Read the model definition and answer for the solid it produces. Units are mm, in the model's axes. A direction names the side the tool comes from. Coordinates: 2 decimals unless noted, no trailing zeros. Loops run counter-clockwise (first coordinate to the right, second up) from the corner with the lowest first, then second, coordinate; pieces in that order, holes last. Notation, with made-up numbers: M 77.25,30.5 L 86.25,30.5 A23 cw 86.25,40.5 Z; hole C -21.75,50 d6. An arc over 180 degrees is marked long. Put each result on its own line as item: value.
Autodesk Inventor part; units mm, degrees
ref_plane "YZ Plane" through (0, 0, 0) normal (1, 0, 0) x (0, 1, 0)
ref_plane "XZ Plane" through (0, 0, 0) normal (0, 1, 0) x (-1, 0, 0)
ref_plane "XY Plane" through (0, 0, 0) normal (0, 0, 1) x (1, 0, 0)
sketch "Sketch1" plane through (0, 0, 0) normal (0, 0, 1) x (1, 0, 0)
  circle A0 centre (-150, 0) radius 225 construction
  line L0 (0, 0) -> (0, 132.2876)
  line L1 (0, 132.2876) -> (17.7086, 149.9961)
  line L2 (0, 132.2876) -> (25.0437, 132.2876) construction
  arc A1 (75, 0) -> (17.7086, 149.9961) centre (-150, 0) ccw
  line L3 (75, 0) -> (25, 0)
  line L4 (25, 0) -> (17.5, 0)
  line L5 (0, 0) -> (7.5, 0)
  line L6 (7.5, 0) -> (7.5, -10)
  line L7 (7.5, -10) -> (17.5, -10)
  line L8 (17.5, -10) -> (17.5, 0)
  circle A2 centre (-150, 0) radius 200 construction
  dimension "d0" = 75
  dimension "d1" = 450
  dimension "d3" = 45
  dimension "d37" = 50
  dimension "d38" = 7.5
  dimension "d39" = 7.5
  dimension "d40" = 10
  dimension "d41" = 25
extrude "Extrusion1" add sketch "Sketch1" along normal blind 15
sketch "Sketch2" plane through (0, 0, 15) normal (0, 0, 1) x (1, 0, 0)
  circle A0 centre (58.5066, 25) radius 2.5
  circle A1 centre (56.1901, 39.8201) radius 2.5
  line L0 (0, 132.2876) -> (0, 0)
  line L1 (0, 0) -> (7.5, 0)
  line L2 (7.5, 0) -> (7.5, -10)
  line L3 (7.5, -10) -> (17.5, -10)
  line L4 (17.5, -10) -> (17.5, 0)
  line L5 (17.5, 0) -> (75, 0)
  arc A2 (75, 0) -> (17.7086, 149.9961) centre (-150, 0) ccw
  line L6 (17.7086, 149.9961) -> (0, 132.2876)
  arc A3 (59.4636, 15) -> (16.6742, 127.7486) centre (-150, 0) ccw construction
  line L7 (59.4636, 15) -> (17.5, 15) construction
  line L8 (17.5, 15) -> (15, 15) construction
  line L9 (15, 15) -> (15, 126.0744) construction
  line L10 (15, 126.0744) -> (16.6742, 127.7486) construction
  circle A4 centre (11.959, 133.676) radius 2.5
  circle A5 centre (-150, 0) radius 225 construction
  circle A6 centre (-150, 0) radius 210 construction
  dimension "d6" = 5
  dimension "d7" = 5
  dimension "d8" = 15
  dimension "d10" = 25
  dimension "d42" = 15
  dimension "d43" = 5
  dimension "d45" = 450
  dimension "d46" = 15
  dimension "d49" = 7.4745
extrude "Extrusion2" cut sketch "Sketch2" against normal through all contours A0 | A1 | A4
sketch "Sketch5" plane through (0, 0, 15) normal (0, 0, 1) x (1, 0, 0)
  line L0 (5, 137.2876) -> (12.0711, 130.2165)
  line L1 (5, 137.2876) -> (15, 137.2876) construction
  line L2 (12.0711, 130.2165) -> (15.6066, 133.752)
  line L3 (15.6066, 133.752) -> (8.5355, 140.8231)
  line L4 (8.5355, 140.8231) -> (5, 137.2876)
  line L5 (17.7086, 149.9961) -> (0, 132.2876)
  point P0 (0, 0)
  dimension "d29" = 10
  dimension "d30" = 45
  dimension "d31" = 5
  dimension "d32" = 10
  dimension "d33" = 90
  dimension "d34" = 5
extrude "Extrusion3" cut sketch "Sketch5" against normal through all
thread "Thread1"
thread "Thread2"
thread "Thread3"
sketch "Sketch6" plane through (0, 0, 15) normal (0, 0, 1) x (1, 0, 0)
  line L0 (0, 107.2876) -> (20, 107.2876) construction
  line L1 (20, 107.2876) -> (20, 57.2876) construction
  line L2 (20, 57.2876) -> (0, 57.2876) construction
  line L3 (0, 57.2876) -> (0, 107.2876) construction
  line L4 (8.5355, 140.8231) -> (15.6066, 133.752) construction
  line L5 (15.6066, 133.752) -> (12.0711, 130.2165) construction
  line L6 (9.7164, 132.5711) -> (5, 137.2876) construction
  line L7 (5, 137.2876) -> (0, 132.2876) construction
  line L8 (0, 132.2876) -> (0, 0) construction
  line L9 (0, 0) -> (7.5, 0) construction
  line L10 (7.5, 0) -> (7.5, -10) construction
  line L11 (7.5, -10) -> (17.5, -10) construction
  line L12 (17.5, -10) -> (17.5, 0) construction
  line L13 (17.5, 0) -> (75, 0) construction
  arc A0 (75, 0) -> (17.7086, 149.9961) centre (-150, 0) ccw construction
  line L14 (17.7086, 149.9961) -> (8.5355, 140.8231) construction
  arc A1 (9.7164, 132.5711) -> (10.8542, 131.4334) centre (11.959, 133.676) ccw construction
  circle A2 centre (58.5066, 25) radius 2.5 construction
  circle A3 centre (56.1901, 39.8201) radius 2.5 construction
  circle A4 centre (10, 92.2876) radius 2.5
  circle A5 centre (10, 72.2876) radius 2.5
  line L15 (0, 132.2876) -> (0, 0)
  line L16 (12.0711, 130.2165) -> (10.8542, 131.4334)
  dimension "d50" = 20
  dimension "d51" = 50
  dimension "d52" = 25
  dimension "d53" = 5
  dimension "d54" = 5
  dimension "d55" = 20
  dimension "d56" = 15
  dimension "d57" = 10
extrude "Extrusion4" cut sketch "Sketch6" against normal through all
thread "Thread4"
thread "Thread5"
sketch "Sketch8" plane through (0, 0, 0) normal (0, 0, -1) x (-1, 0, 0)
  line L0 (0, 132.2876) -> (0, 0)
  line L1 (0, 107.2876) -> (-20, 107.2876)
  line L2 (-20, 107.2876) -> (-20, 57.2876)
  line L3 (-20, 57.2876) -> (0, 57.2876)
  line L4 (0, 57.2876) -> (0, 107.2876)
  dimension "d69" = 20
  dimension "d70" = 50
  dimension "d71" = 25
extrude "Extrusion6" cut sketch "Sketch8" against normal blind 5
properties part number "CP001" material "ABS Plastic"
1) Find section D-D, the plane x = 51.5. Write down the section's boundary in (y, z).
Answer list:
outline: M 0,0 L 100.11,0 L 100.11,15 L 0,15 Z
2) Given pin 1 Ø2.5 at (x, z) = (5.5, 2.5) entering from -Y; pin 2 Ø4 at (x, y) = (10, 72.29) entering from +Z; pin 3 Ø2 at (x, z) = (55.5, 7.5) entering from +Y; pin 4 Ø2.5 at (y, z) = (81.5, 3.5) entering from -X, each flat-ended and moving along its own axis, determine where each tip first touches the part or whether it passes through.
Answer list:
pin 1: stops at y = 0
pin 2: passes through
pin 3: stops at y = 93.83
pin 4: stops at x = 20
3) Find section A-A, the plane y = 25. Write down the section's boundary in (x, z), plus the area to 3 significant figures.
Answer list:
outline: M 0,0 L 56.01,0 L 56.01,15 L 0,15 Z; M 61.01,0 L 73.61,0 L 73.61,15 L 61.01,15 Z
area: 1,030 mm^2
4) Find section B-B, the plane z = 2.25. Write down the section's boundary in (x, y).
Answer list:
outline: M 0,0 L 7.5,0 L 7.5,-10 L 17.5,-10 L 17.5,0 L 75,0 A225 ccw 17.71,150 L 8.54,140.82 L 15.61,133.75 L 12.07,130.22 L 10.85,131.43 A2.5 cw 9.72,132.57 L 5,137.29 L 0,132.29 L 0,107.29 L 20,107.29 L 20,57.29 L 0,57.29 Z; hole C 56.19,39.82 d5; hole C 58.51,25 d5
5) Find section C-C, the plane z = 9.25. Write down the section's boundary in (x, y).
Answer list:
outline: M 0,0 L 7.5,0 L 7.5,-10 L 17.5,-10 L 17.5,0 L 75,0 A225 ccw 17.71,150 L 8.54,140.82 L 15.61,133.75 L 12.07,130.22 L 10.85,131.43 A2.5 cw 9.72,132.57 L 5,137.29 L 0,132.29 Z; hole C 10,72.29 d5; hole C 10,92.29 d5; hole C 56.19,39.82 d5; hole C 58.51,25 d5
6) Determine the mould class of faces 6 (the flat face through (37, 53, 0)), 7 (the flat face through (7.33, 134.96, 7.6)), 8 (the flat face through (13.06, 145.35, 7.4)), 9 (the cylindrical face through (9.458, 69.847, 10.07)) for opening direction X: released by +X, released by -X, zero draft, split by the parting line, or undercut.
Answer list:
face 6: zero draft
face 7: undercut
face 8: released by -X
face 9: undercut
7) Which of the six approach directions +Z, -Z, +X, -X, +Y, -Y give full straight-line access (tool end or side, diameter ignored) to faces 1 (the flat face through (13.814, 131.96, 7.605)), 2 (the flat face through (4, 0, 7)), 3 (the flat face through (10, 57.288, 2)), 4 (the flat face through (2.465, 134.753, 7.395)), 5 (the flat face through (17.5, -5, 7))?
Answer list:
face 1: +Z, -Z
face 2: +Z, -Z, -X, -Y
face 3: -Z, -X
face 4: +Z, -Z, -X, +Y
face 5: +Z, -Z, +X, -Y
8) Straight lines are drawn through the part: line 1 (Y direction, x = 10, z = 12); line 2 (X direction, y = 24.5, z = 1); line 3 (X direction, y = 39, z = 6). For each, find the intervals that lie inside material, in ascending order. Write a range as [from, to].
Answer list:
line 1: y = [-10, 69.79], [74.79, 89.79], [94.79, 132.12], [139.36, 142.29]
line 2: x = [0, 56.06], [60.96, 73.66]
line 3: x = [0, 53.83], [58.55, 71.59]
